Source: CAD feature listing. Evaluate the final solid. Frame: model axes, mm. Round coordinates to 2 decimals unless told otherwise and drop trailing zeros. Order: outer loops, then holes, each group sorted by start corner. A loop starts at its lowest first (then second) coordinate and runs counter-clockwise, first axis right, second up. Notation, with made-up numbers: (51, 88) -> (89, 88) arc R20 cw to (89, 92) -> close; hole circle Ø10 at (-1, 24). An arc over 180 degrees is marked (long way). Use a Markdown table: item, result. Add a question column.
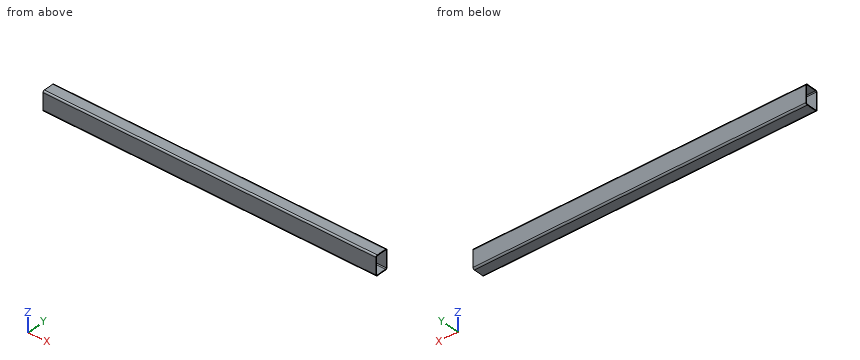
```python
from build123d import *

# Parameters (mm, degrees)
F0_W     = 50
F0_H     = 75
F1_DEPTH = 1280
F2_R     = 6
F3_T     = -3


with BuildPart() as f1:
    # F0 (on Right) → F1 (new body)
    with BuildSketch(Plane.YZ):
        Rectangle(F0_W, F0_H)
    extrude(amount=F1_DEPTH)

    # F2
    f2_edges = [f1.edges().sort_by_distance(p)[0] for p in [
        (640, 25, 37.5),
        (640, -25, 37.5),
        (640, 25, -37.5),
        (640, -25, -37.5),
    ]]
    fillet(f2_edges, radius=F2_R)

    # F3
    f3_openings = [f1.faces().sort_by_distance(p)[0] for p in [
        (0, 0, 0),
        (1280, 0, 0),
    ]]
    offset(amount=F3_T, openings=f3_openings)


solid = f1.part
```
1) Section B-B on x = 676. Output: boundary loops of the cut face in (y, z).
2) Section A-A on y = -4. Output: boundary loops of the cut face in (x, z), then the cut area to 3 significant figures.
3) Line query: probe 1 along Y at (x, z) = (459, 32.5); probe 2 along Z at (x, y) = (693, 4); probe 3 along Y at (x, z) = (1060.5, 13.5). Output: solid intervals per line, ascending. Write a range as from..to.
4) Section C-C on z = 16. Output: boundary loops of the cut face in (x, y), then the cut area to 3 significant figures.
Conclusion:
| question | item | result |
|---|---|---|
| 1 | outline | (-25, -31.5) arc R6 ccw to (-19, -37.5) -> (19, -37.5) arc R6 ccw to (25, -31.5) -> (25, 31.5) arc R6 ccw to (19, 37.5) -> (-19, 37.5) arc R6 ccw to (-25, 31.5) -> close; hole (-22, -31.5) arc R3 ccw to (-19, -34.5) -> (19, -34.5) arc R3 ccw to (22, -31.5) -> (22, 31.5) arc R3 ccw to (19, 34.5) -> (-19, 34.5) arc R3 ccw to (-22, 31.5) -> close |
| 2 | outline | (0, -37.5) -> (1280, -37.5) -> (1280, -34.5) -> (0, -34.5) -> close; (0, 34.5) -> (1280, 34.5) -> (1280, 37.5) -> (0, 37.5) -> close |
| 2 | area | 7,680 mm^2 |
| 3 | probe 1 | y = -24.92..-21.83, 21.83..24.92 |
| 3 | probe 2 | z = -37.5..-34.5, 34.5..37.5 |
| 3 | probe 3 | y = -25..-22, 22..25 |
| 4 | outline | (0, -25) -> (1280, -25) -> (1280, -22) -> (0, -22) -> close; (0, 22) -> (1280, 22) -> (1280, 25) -> (0, 25) -> close |
| 4 | area | 7,680 mm^2 |
